```python
from build123d import *

# Parameters (mm, degrees)
BOSS_EXTRU_1_DEPTH      = 10
ESQUISSE2_W             = 49.45
ESQUISSE2_H             = 24.53
BOSS_EXTRU_2_DEPTH      = 2
ESQUISSE3_R             = 1
ENL_V_MAT_EXTRU_1_DEPTH = 2
ESQUISSE7_W             = 49.45
ESQUISSE7_H             = 30
BOSS_EXTRU_3_DEPTH      = 2
ESQUISSE8_R             = 1.5
ENL_V_MAT_EXTRU_2_DEPTH = 2


with BuildPart() as part:
    # Esquisse1 → Boss.-Extru.1 (new body)
    with BuildSketch(Plane.XY):
        Polygon((8.740819068, -15.001789588), (26.465819068, -15.001789588), (26.465819068, 9.528210412), (-22.984180932, 9.528210412), (-22.984180932, -15.001789588), (-5.259180932, -15.001789588), (-5.259180932, -13.001789588), (-20.984180932, -13.001789588), (-20.984180932, 7.528210412), (24.465819068, 7.528210412), (24.465819068, -13.001789588), (8.740819068, -13.001789588), align=None)
    extrude(amount=BOSS_EXTRU_1_DEPTH)

    # Esquisse2 → Boss.-Extru.2 (add)
    with BuildSketch(Plane(origin=(0, 0, 0), x_dir=(-1, 0, 0), z_dir=(0, 0, -1))):
        with Locations((-1.740819068, -2.736789588)):
            Rectangle(ESQUISSE2_W, ESQUISSE2_H)
    extrude(amount=BOSS_EXTRU_2_DEPTH)

    # Esquisse3 → Enlèv. mat.-Extru.1 (cut)
    with BuildSketch(Plane.XY):
        with Locations((-19.384180932, -11.401789588)):
            Circle(ESQUISSE3_R)
        with Locations(Location((22.865819068, -11.401789588, 0), (0, 0, 180))):
            Circle(ESQUISSE3_R)
        with Locations((22.865819068, 5.928210412)):
            Circle(ESQUISSE3_R)
        with Locations(Location((-19.384180932, 5.928210412, 0), (0, 0, 180))):
            Circle(ESQUISSE3_R)
    extrude(amount=-ENL_V_MAT_EXTRU_1_DEPTH, mode=Mode.SUBTRACT)

    # Esquisse7 → Boss.-Extru.3 (add)
    with BuildSketch(Plane(origin=(0, 9.528210412, 0), x_dir=(1, 0, 0), z_dir=(0, 1, 0))):
        with Locations((1.740819068, 5)):
            Rectangle(ESQUISSE7_W, ESQUISSE7_H)
    extrude(amount=BOSS_EXTRU_3_DEPTH)

    # Esquisse8 → Enlèv. mat.-Extru.2 (cut)
    with BuildSketch(Plane(origin=(0, 11.528210412, 0), x_dir=(1, 0, 0), z_dir=(0, 1, 0))):
        with Locations(Location((-15.484180932, 12.5, 0), (0, 0, 180))):
            Circle(ESQUISSE8_R)
        with Locations((18.965819068, 12.5)):
            Circle(ESQUISSE8_R)
    extrude(amount=-ENL_V_MAT_EXTRU_2_DEPTH, mode=Mode.SUBTRACT)


solid = part.part
```
CAD build for the part. Positions are in the model's coordinates, mm. A direction names the side the tool comes from. Round coordinates to 2 decimals unless told otherwise and drop trailing zeros. Order: outer loops, then holes, each group sorted by start corner. A loop starts at its lowest first (then second) coordinate and runs counter-clockwise, first axis right, second up. Notation, with made-up numbers: (-0.75, -22.75) - (23.25, -22.75) arc R11 cw to (23.25, -10.75) - close; hole circle Ø8 at (87, 40). An arc over 180 degrees is marked (long way). Use CSV: the item, a comma, the result in double quotes. Start each with the question number.
1) Pin check, flat tips, straight feed: pin 1 Ø1.8 at (x, y) = (22.87, 5.93) entering from -Z; pin 2 Ø1.5 at (x, y) = (18, -3.5) entering from +Z; pin 3 Ø10 at (x, z) = (-10, -10.5) entering from -Y; pin 4 Ø6 at (x, y) = (-5.5, -12) entering from -Z. Stop position of each tip, or through.
2) Saw through at A-A (z = -12.5). List the corners of the cut face in (x, y).
3) Tool access for faces 1 (the flat face through (-5.259, -14, 5)), 2 (the flat face through (2, -3, -2)), 3 (the flat face through (24.466, -3, 5)), 4 (the flat face through (2, 9, 10)): list every direction of +Z, -Z, +X, -X, +Y, -Y with a clear straight run to the whole face (end or side of a thin tool).
4) Two-plate mould, pull along Z, no slides. Class faces 5 (the flat face through (1, 11, -20)), 6 (the cylindrical face through (-16.9, 10.5, -12)), 7 (the flat face through (8.741, -14, 5)): pulls with the +Z half, pulls with the -Z half, needs draft (parallel to the pull), parting line crosses it, or undercut.
5) Saw through at C-C (y = -5). List the corners of the cut face in (x, z).
6) Saw through at B-B (x = -8). List the corners of the cut face in (y, z), and give its area (3 significant figures).
7) Saw through at D-D (z = 6.5). List the corners of the cut face in (x, y).
8) Wall check: L1, parallel to Y at x = -16.5, z = 2.5; L2, parallel to X at y = 7, z = 2.75; L3, parallel to Y at x = 9, z = -17.5. Give the ranges that are in metal, low to high. Write a range as [from, to].
Values follow:
1,pin 1,"passes through"
1,pin 2,"stops at z = 0"
1,pin 3,"stops at y = 9.53"
1,pin 4,"stops at z = -2"
2,outline,"(-22.98, 9.53) - (-16.98, 9.53) - (-16.98, 11.53) - (-22.98, 11.53) - close; (-13.98, 9.53) - (17.47, 9.53) - (17.47, 11.53) - (-13.98, 11.53) - close; (20.47, 9.53) - (26.47, 9.53) - (26.47, 11.53) - (20.47, 11.53) - close"
3,face 1,"+Z, -Y"
3,face 2,"-Z, +X, -X, -Y"
3,face 3,"+Z"
3,face 4,"+Z, +X, -X, +Y, -Y"
4,face 5,"pulls with the -Z half"
4,face 6,"undercut"
4,face 7,"needs draft"
5,outline,"(-22.98, -2) - (26.47, -2) - (26.47, 10) - (24.47, 10) - (24.47, 0) - (-20.98, 0) - (-20.98, 10) - (-22.98, 10) - close"
6,outline,"(-15, -2) - (9.53, -2) - (9.53, -20) - (11.53, -20) - (11.53, 10) - (7.53, 10) - (7.53, 0) - (-13, 0) - (-13, 10) - (-15, 10) - close"
6,area,"149 mm2"
7,outline,"(-22.98, -15) - (-5.26, -15) - (-5.26, -13) - (-20.98, -13) - (-20.98, 7.53) - (24.47, 7.53) - (24.47, -13) - (8.74, -13) - (8.74, -15) - (26.47, -15) - (26.47, 11.53) - (-22.98, 11.53) - close"
8,L1,"y = [-15, -13], [7.53, 11.53]"
8,L2,"x = [-22.98, -20.98], [24.47, 26.47]"
8,L3,"y = [9.53, 11.53]"
